Can you work these out from the model? Positions are in its coordinate system, mm. Face numbers are marked on the shaded views. Give positions to 0.01 mm unless a question says otherwise; leave off trailing zeros. Loops run counter-clockwise (first coordinate to the right, second up) from the corner with the lowest first, then second, coordinate; pieces in that order, holes last. Notation, with made-up numbers: (-11, 81.25) - (23, 81.25) arc R15 cw to (23, 108.25) - close; hole circle Ø9 at (-28.5, 5.25). An arc over 180 degrees is marked (long way). Write item = value, one per line.
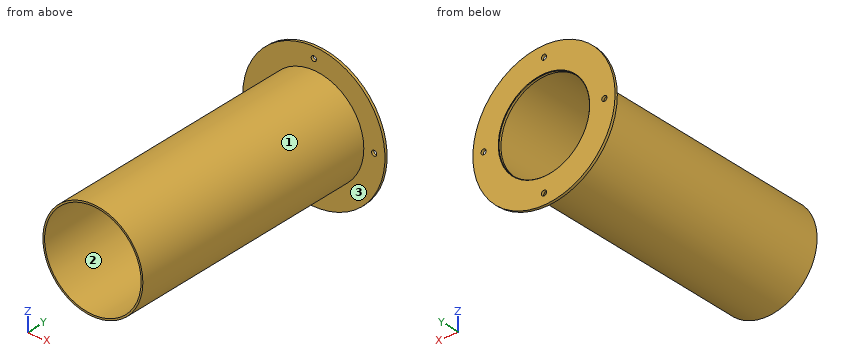
Autodesk Inventor part; units mm, degrees
ref_plane "YZ Plane" through (0, 0, 0) normal (1, 0, 0) x (0, 1, 0)
ref_plane "XZ Plane" through (0, 0, 0) normal (0, 1, 0) x (-1, 0, 0)
ref_plane "XY Plane" through (0, 0, 0) normal (0, 0, 1) x (1, 0, 0)
sketch "Sketch1" plane through (0, 0, 0) normal (0, 1, 0) x (-1, 0, 0)
  circle A0 centre (0, 0) radius 52.5
  circle A1 centre (0, 0) radius 82.5
  dimension "d1" = 105
  dimension "d2" = 30
extrude "Extrusion1" add sketch "Sketch1" along normal blind 3
chamfer "Chamfer1" distance 0.5 angle 45 1 edges at (52.5, 3, 0)
sketch "Sketch4" plane through (0, 0, 0) normal (0, -1, 0) x (1, 0, 0)
  circle A0 centre (0, 0) radius 70 construction
  circle A1 centre (0, 70) radius 3
  circle A2 centre (-70, 0) radius 3
  circle A3 centre (0, -70) radius 3
  circle A4 centre (70, 0) radius 3
  dimension "d14" = 140
  dimension "d15" = 6
  dimension "d18" = 360
hole "Hole1" at (0, 0, 70) at (70, 0, 0) at (0, 0, -70) at (-70, 0, 0) direction (0, 1, 0) diameter 6 end through all
sketch "Sketch5" plane through (0, 0, 0) normal (0, -1, 0) x (1, 0, 0)
  circle A0 centre (0, 0) radius 56
  circle A1 centre (0, 0) radius 58
  dimension "d28" = 112
  dimension "d29" = 116
extrude "Extrusion3" add sketch "Sketch5" along normal blind 300
properties part number "110mm_flange"
Q1. Imagine slicing it at A-A, the plane y = -268.5. Write out the boundary of the cut face in (x, z), then the cut area to 3 significant figures.
Output:
outline = circle Ø116 at (0, 0); hole circle Ø112 at (0, 0)
area = 716 mm2
Q2. I need wall thicknesses on L1, parallel to Z at x = 0, y = 1.75; L2, parallel to Z at x = 2, y = -94.5; L3, parallel to Y at x = 47.5, z = -51. Which ranges of each line are inside material? Lowest first, please.
Output:
L1 = -82.5 to -73, -67 to -52.5, 52.5 to 67, 73 to 82.5
L2 = -57.97 to -55.96, 55.96 to 57.97
L3 = 0 to 3
Q3. We'd pull the mould along Z, two halves only. Please class the marked faces 1, 2 and 3: released by +Z, released by -Z, zero draft, split by the parting line, or undercut.
Output:
face_1 = split by the parting line
face_2 = undercut
face_3 = zero draft
Q4. For pin 1 (1 mm diameter, centred on y = -236.5, z = 29, fed in from -X); pin 2 (12 mm diameter, centred on x = 35, y = -204.5, fed in from +Z); pin 3 (2 mm diameter, centred on y = -118.5, z = 26, fed in from +X), each with a flat end and sliding along its axis, tell me the tip position at first contact or that it passes through.
Output:
pin_1 = -50.51
pin_2 = 50.23
pin_3 = 52.34
